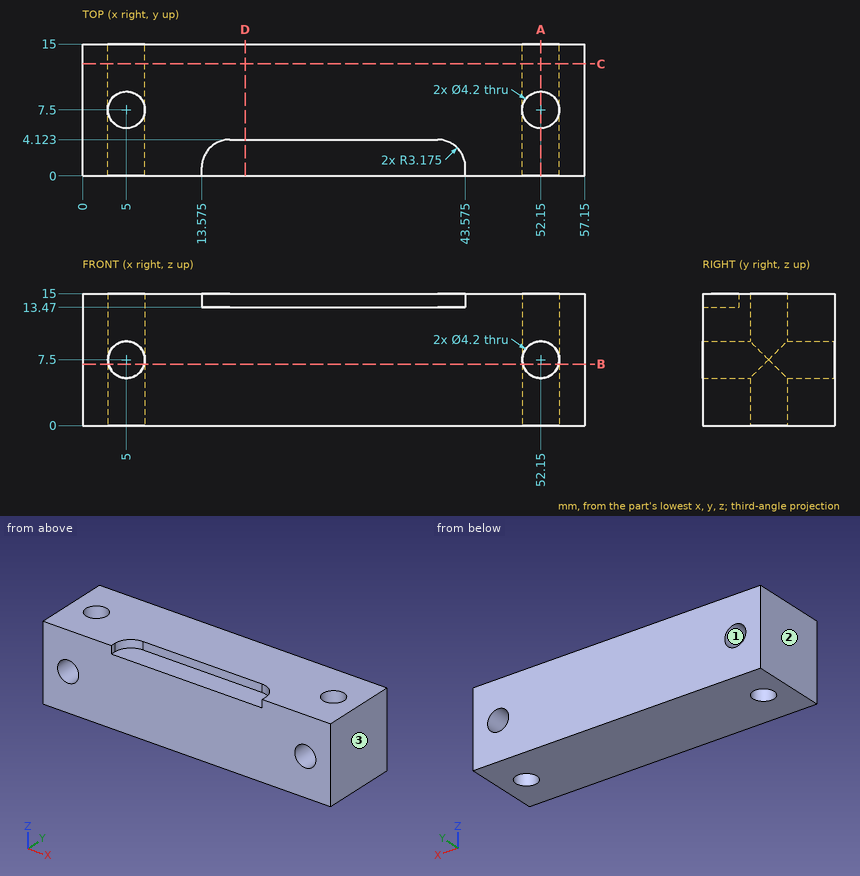
Here's the drawing with two shaded views (mm, measured from the low corner). I have some questions. Coordinates: 2 decimals unless noted, no trailing zeros. Loops run counter-clockwise (first coordinate to the right, second up) from the corner with the lowest first, then second, coordinate; pieces in that order, holes last. Notation, with made-up numbers: (69.5, 81) -> (86.5, 81) arc R8 cw to (86.5, 88) -> close; hole circle Ø7 at (34.5, -2.5). An arc over 180 degrees is marked (long way). Answer in a Markdown table with one row per item.
(1) Imagine slicing it at C-C (y = 12.75). List the corners of the cut face in (x, z) for me.
Results found:
| item | result |
|---|---|
| outline | (0, 0) -> (57.15, 0) -> (57.15, 15) -> (0, 15) -> close; hole circle Ø4.2 at (5, 7.5); hole circle Ø4.2 at (52.15, 7.5) |
(2) Imagine slicing it at B-B (z = 7). List the corners of the cut face in (x, y) for me, plus the area to 3 significant figures.
Results found:
| item | result |
|---|---|
| outline | (0, 0) -> (2.96, 0) -> (2.96, 7) arc R2.1 cw to (2.96, 8) -> (2.96, 15) -> (0, 15) -> close; (7.04, 0) -> (50.11, 0) -> (50.11, 7) arc R2.1 cw to (50.11, 8) -> (50.11, 15) -> (7.04, 15) -> (7.04, 8) arc R2.1 cw to (7.04, 7) -> close; (54.19, 0) -> (57.15, 0) -> (57.15, 15) -> (54.19, 15) -> (54.19, 8) arc R2.1 cw to (54.19, 7) -> close |
| area | 735 mm^2 |
(3) Thinking about a two-plate mould opening in X: for the marked faces 1, 2 and 3, which applies, released by +X, released by -X, zero draft, split by the parting line, or undercut?
Results found:
| item | result |
|---|---|
| face 1 | undercut |
| face 2 | released by -X |
| face 3 | released by +X |
(4) Imagine slicing it at D-D (x = 18.5). List the corners of the cut face in (y, z) for me.
Results found:
| item | result |
|---|---|
| outline | (0, 0) -> (15, 0) -> (15, 15) -> (4.12, 15) -> (4.12, 13.47) -> (0, 13.47) -> close |
(5) If I drill on probe 1 along X at (y, z) = (7.5, 13.5); probe 2 along X at (y, z) = (8, 4.5); probe 3 along Z at (x, y) = (5, 2.25), over which ranges is the centre line in solid material (lowest first)?
Results found:
| item | result |
|---|---|
| probe 1 | x = 0 to 2.9, 7.1 to 50.05, 54.25 to 57.15 |
| probe 2 | x = 0 to 2.96, 7.04 to 50.11, 54.19 to 57.15 |
| probe 3 | z = 0 to 5.4, 9.6 to 15 |
(6) Imagine slicing it at A-A (x = 52.15). List the corners of the cut face in (y, z) for me.
Results found:
| item | result |
|---|---|
| outline | (0, 0) -> (5.4, 0) -> (5.4, 5.4) -> (0, 5.4) -> close; (0, 9.6) -> (5.4, 9.6) -> (5.4, 15) -> (0, 15) -> close; (9.6, 0) -> (15, 0) -> (15, 5.4) -> (9.6, 5.4) -> close; (9.6, 9.6) -> (15, 9.6) -> (15, 15) -> (9.6, 15) -> close |
(7) Will these pins go through, and if not, where does the flat tip stop? pin 1 Ø0.5 at (x, z) = (32, 14.5) entering from -Y; pin 2 Ø2 at (x, y) = (32, 1.5) entering from +Z.
Results found:
| item | result |
|---|---|
| pin 1 | stops at y = 4.12 |
| pin 2 | stops at z = 13.47 |
